Part model, mm, in its own coordinate system. A direction names the side the tool comes from. Coordinates: 2 decimals unless noted, no trailing zeros. Loops run counter-clockwise (first coordinate to the right, second up) from the corner with the lowest first, then second, coordinate; pieces in that order, holes last. Notation, with made-up numbers: (38, -14) -> (83, -14) arc R28 cw to (83, 25) -> close; hole circle Ø3 at (56, -14). An arc over 180 degrees is marked (long way). One line per question, with ' | ' between items. Start each with the question number.
1) Cut at C-C (z = 25.5). List the corners of the cut face in (x, y), plus the area to 3 significant figures.
2) Cut at B-B (y = 11). List the corners of the cut face in (x, z).
3) 3-axis set-ups, long thin cutter, end or side, ignore diameter. For faces 1 (the face through (48.034, 9.86, 25.219)), 2 (the face through (30.086, 10, 39)), 3 (the face through (40.086, 10, 39)): which of +Z, -Z, +X, -X, +Y, -Y reach the whole face in a straight line?
4) Probe L1, parallel to X at y = 1.5, z = 37.75; L2, parallel to X at y = 1.5, z = 27.5; L3, parallel to Z at x = 35, y = 9.25. List the from-to ranges inside material, lowest first. Write a range as from..to.
5) Drop flat-ended pins along their axis: pin 1 (4 mm diameter, centred on y = 12.5, z = 32, fed in from +X); pin 2 (3.5 mm diameter, centred on y = 6.5, z = 39, fed in from +X); pin 3 (7.5 mm diameter, centred on y = 11, z = 38, fed in from -X). Give the stop position or say it passes through.
6) Cut at A-A (z = 29.25). List the corners of the cut face in (x, y).
7) Cut at D-D (x = 35.5). List the corners of the cut face in (y, z), plus the area to 3 significant figures.
from build123d import *

# Parameters (mm, degrees)
F1_DEPTH = 20


with BuildPart() as f1:
    # F0 (on Front) → F1 (new body)
    with BuildSketch(Plane.XZ):
        with BuildLine():
            Line((19.2999951541, 26.6305115074), (24.9214912266, 23.8985655014))
            ThreePointArc((24.9214912266, 23.8985655014), (29.0725771912, 28.5851222957), (35.0859551343, 30.32713693))
            Line((35.0859551343, 30.32713693), (30.0859551343, 30.32713693))
            Line((30.0859551343, 30.32713693), (30.0859551343, 35.8476467612))
            ThreePointArc((30.0859551343, 35.8476467612), (23.7170093324, 32.38116156), (19.2999951541, 26.6305115074))
        make_face()
        with BuildLine():
            Line((30.0859551343, 30.32713693), (35.0859551343, 30.32713693))
            Line((35.0859551343, 30.32713693), (40.0859551343, 30.32713693))
            Line((40.0859551343, 30.32713693), (40.0859551343, 35.8476467612))
            ThreePointArc((40.0859551343, 35.8476467612), (35.0859551343, 36.57713693), (30.0859551343, 35.8476467612))
            Line((30.0859551343, 35.8476467612), (30.0859551343, 30.32713693))
        make_face()
        with BuildLine():
            Line((30.0859551343, 42.82713693), (30.0859551343, 35.8476467612))
            ThreePointArc((30.0859551343, 35.8476467612), (35.0859551343, 36.57713693), (40.0859551343, 35.8476467612))
            Line((40.0859551343, 35.8476467612), (40.0859551343, 42.82713693))
            Line((40.0859551343, 42.82713693), (30.0859551343, 42.82713693))
        make_face()
        with BuildLine():
            Line((40.0859551343, 30.32713693), (35.0859551343, 30.32713693))
            ThreePointArc((35.0859551343, 30.32713693), (41.0993330773, 28.5851222957), (45.2504190419, 23.8985655014))
            Line((45.2504190419, 23.8985655014), (50.8973434351, 26.57713693))
            ThreePointArc((50.8973434351, 26.57713693), (46.477357984, 32.3619380619), (40.0859551343, 35.8476467612))
            Line((40.0859551343, 35.8476467612), (40.0859551343, 30.32713693))
        make_face()
    extrude(amount=-F1_DEPTH)


solid = f1.part
Reported:
1) outline: (21.63, 0) -> (25.85, 0) -> (25.85, 20) -> (21.63, 20) -> close; (44.32, 0) -> (48.63, 0) -> (48.63, 20) -> (44.32, 20) -> close | area: 171 mm²
2) outline: (19.3, 26.63) -> (24.92, 23.9) arc R11.25 cw to (45.25, 23.9) -> (50.9, 26.58) arc R17.5 ccw to (40.09, 35.85) -> (40.09, 42.83) -> (30.09, 42.83) -> (30.09, 35.85) arc R17.5 ccw to start
3) face 1: -Z, +X, +Y, -Y | face 2: +Z, -X, +Y, -Y | face 3: +Z, +X, +Y, -Y
4) L1: x = 30.09..40.09 | L2: x = 19.75..27.63, 42.54..50.43 | L3: z = 30.33..42.83
5) pin 1: stops at x = 48.76 | pin 2: stops at x = 40.09 | pin 3: stops at x = 26.37
6) outline: (20.85, 0) -> (30.28, 0) -> (30.28, 20) -> (20.85, 20) -> close; (39.89, 0) -> (49.33, 0) -> (49.33, 20) -> (39.89, 20) -> close
7) outline: (0, 30.32) -> (20, 30.32) -> (20, 42.83) -> (0, 42.83) -> close | area: 250 mm²
